from build123d import *

# Parameters (mm, degrees)
F1_DEPTH = 50.8
F3_DEPTH = 114.3


with BuildPart() as f1:
    # F0 (on Right) → F1 (new body)
    with BuildSketch(Plane.YZ):
        Polygon((-52.681003, -18.723272), (-39.981003, -18.723272), (48.918997, -18.723272), (48.918997, 32.076728), (36.218997, 32.076728), (36.218997, -6.023272), (-39.981003, -6.023272), (-39.981003, 32.076728), (-52.681003, 32.076728), align=None)
    extrude(amount=F1_DEPTH)

    # F2 (on face) → F3 (cut, symmetric)
    with BuildSketch(Plane.XZ.offset(52.681003)):
        Polygon((24.353357, 0.326728), (38.1, 0.326728), (38.1, 13.026728), (38.1, 25.726728), (25.4, 25.726728), (12.7, 25.726728), (12.7, 9.816655), (12.7, 0.326728), align=None)
    extrude(amount=F3_DEPTH, both=True, mode=Mode.SUBTRACT)


solid = f1.part
Geometry check sheet. Reference: the model listing, model coordinates, mm. A direction names the side the tool comes from. Round coordinates to 2 decimals unless told otherwise and drop trailing zeros. Loops run counter-clockwise (first coordinate to the right, second up) from the corner with the lowest first, then second, coordinate; pieces in that order, holes last. Notation, with made-up numbers: (76, -34.75) -> (110, -34.75) arc R11 cw to (110, -26.75) -> close; hole circle Ø8 at (30.5, 84.5). An arc over 180 degrees is marked (long way). Answer as a JSON object with one key per item and string values. Group by question number.
Item 1: Thickness scan on line 1 along Z through (x, y) = (24, -44); line 2 along Y through (x, z) = (12, 22.5); line 3 along X through (y, z) = (-44, 1.5). Record the ranges inside material, lowest first.
Item 2: Release check for a two-part mould opening along Z. For faces 4 (the face through (25, 36.219, 26)), 5 (the face through (25, -1, -6.023)), 6 (the face through (26, 42, 25.727)) record: pulls with the +Z half, pulls with the -Z half, needs draft (parallel to the pull), parting line crosses it, or undercut.
Item 3: Cross-section at C-C, the plane x = 7. Record the cut outline in (y, z), plus the area to 3 significant figures.
Item 4: Cross-section at D-D, the plane z = -3.5. Record the cut outline in (x, y).
Item 5: Set-up check for faces 1 (the face through (25, -46, 0.327)), 2 (the face through (0, -3, -10)), 3 (the face through (25, -39.981, 0)): record each of +Z, -Z, +X, -X, +Y, -Y from which the full face is reachable in a straight line by a thin tool's end or side.
Item 6: Cross-section at B-B, the plane z = 22. Record the cut outline in (x, y), plus the area to 3 significant figures.
Item 7: Cross-section at A-A, the plane y = -46. Record the cut outline in (x, z).
Item 8: Depth check by flat-ended pin: pin 1 Ø12 at (x, y) = (10, 11) entering from +Z. Enter the tip coordinate at first touch or a pass-through.
Determined:
{
 "1": {"line 1": "z = -18.72 to 0.33, 25.73 to 32.08", "line 2": "y = -52.68 to -39.98, 36.22 to 48.92", "line 3": "x = 0 to 12.7, 38.1 to 50.8"},
 "2": {"face 4": "needs draft", "face 5": "pulls with the +Z half", "face 6": "undercut"},
 "3": {"outline": "(-52.68, -18.72) -> (48.92, -18.72) -> (48.92, 32.08) -> (36.22, 32.08) -> (36.22, -6.02) -> (-39.98, -6.02) -> (-39.98, 32.08) -> (-52.68, 32.08) -> close", "area": "2,260 mm²"},
 "4": {"outline": "(0, -52.68) -> (50.8, -52.68) -> (50.8, -39.98) -> (0, -39.98) -> close; (0, 36.22) -> (50.8, 36.22) -> (50.8, 48.92) -> (0, 48.92) -> close"},
 "5": {"face 1": "+Y, -Y", "face 2": "+Z, -Z, -X, +Y, -Y", "face 3": "+Z, +X, -X"},
 "6": {"outline": "(0, -52.68) -> (12.7, -52.68) -> (12.7, -39.98) -> (0, -39.98) -> close; (0, 36.22) -> (12.7, 36.22) -> (12.7, 48.92) -> (0, 48.92) -> close; (38.1, -52.68) -> (50.8, -52.68) -> (50.8, -39.98) -> (38.1, -39.98) -> close; (38.1, 36.22) -> (50.8, 36.22) -> (50.8, 48.92) -> (38.1, 48.92) -> close", "area": "645 mm²"},
 "7": {"outline": "(0, -18.72) -> (50.8, -18.72) -> (50.8, 32.08) -> (0, 32.08) -> close; hole (12.7, 0.33) -> (38.1, 0.33) -> (38.1, 25.73) -> (12.7, 25.73) -> close"},
 "8": {"pin 1": "stops at z = -6.02"}
}
